Geometry check sheet. Reference: the model listing, model coordinates, mm. A direction names the side the tool comes from. Coordinates: 2 decimals unless noted, no trailing zeros. Loops run counter-clockwise (first coordinate to the right, second up) from the corner with the lowest first, then second, coordinate; pieces in that order, holes last. Notation, with made-up numbers: (-9, 30.25) - (2, 30.25) arc R27 ccw to (2, 54.25) - close; hole circle Ø6 at (87, 86.5). An arc over 180 degrees is marked (long way). Write item = value, one per line. Start each with the question number.
from build123d import *

# Parameters (mm, degrees)
SKETCH1_W              = 15
SKETCH1_H              = 15
SKETCH1_W_2            = 12
SKETCH1_H_2            = 12
EXTRUDE_THIN1_DEPTH    = 235
CUT_EXTRUDE1_OUTLINE_R = 1.5
CUT_EXTRUDE1_DEPTH     = 15
SKETCH3_R              = 1.5
CUT_EXTRUDE2_DEPTH     = 236.95550428


# Read off the part's stored shape, not the designer's step: Cut-Extrude1
with BuildPart() as part:
    # Sketch1 → Extrude-Thin1 (new body)
    with BuildSketch(Plane(origin=(0, 0, 0), x_dir=(1, 0, 0), z_dir=(0, 1, 0))):
        with Locations((7.5, 7.5)):
            Rectangle(SKETCH1_W, SKETCH1_H)
        with Locations((7.5, 7.5)):
            Rectangle(SKETCH1_W_2, SKETCH1_H_2, mode=Mode.SUBTRACT)
    extrude(amount=EXTRUDE_THIN1_DEPTH)

    # Cut-Extrude1 outline → Cut-Extrude1 (cut)
    with BuildSketch(Plane.YZ):
        with Locations((15, -7.5)):
            Circle(CUT_EXTRUDE1_OUTLINE_R)
        with Locations((5, -7.5)):
            Circle(CUT_EXTRUDE1_OUTLINE_R)
        with Locations((220, -7.5)):
            Circle(CUT_EXTRUDE1_OUTLINE_R)
        with Locations((230, -7.5)):
            Circle(CUT_EXTRUDE1_OUTLINE_R)
    extrude(amount=CUT_EXTRUDE1_DEPTH, mode=Mode.SUBTRACT)

    # Sketch3 → Cut-Extrude2 (cut, through all)
    with BuildSketch(Plane(origin=(15, 0, 0), x_dir=(0, 0, -1), z_dir=(1, 0, 0))):
        with Locations((7.5, 80)):
            Circle(SKETCH3_R)
        with Locations((7.5, 70)):
            Circle(SKETCH3_R)
    extrude(amount=-CUT_EXTRUDE2_DEPTH, mode=Mode.SUBTRACT)


solid = part.part
(1) Sectioned sample at C-C on x = 10. Enter the section's corners in (y, z), plus the area to 3 significant figures.
(2) Tool access check on faces 1 (the face through (0, 116, -7)), 2 (the face through (7, 116, -1.5)). Record the directions out of +Z, -Z, +X, -X, +Y, -Y that give a thin tool (end or side, any length) a straight path to the whole face; none if there is none.
(3) Scan lines: line 1 (X direction, y = 50, z = -3.5); line 2 (Z direction, x = 13.95, y = 80); line 3 (Z direction, x = 2.5, y = 218.5). Record each from-to range of solid material in increasing order.
(4) Draft check along Z on faces 3 (the face through (13.5, 116, -7)), 4 (the face through (15, 116, -7)), 5 (the face through (7, 116, -15)), 6 (the face through (7, 116, 0)). Enter one of: pulls with the +Z half, pulls with the -Z half, needs draft (parallel to the pull), parting line crosses it, or undercut.
(5) Sectioned sample at A-A on z = -11. Enter the section's corners in (x, y).
(6) Sectioned sample at B-B on y = 96. Enter the section's corners in (x, z).
Working result:
q1.outline = (0, -15) - (235, -15) - (235, -13.5) - (0, -13.5) - close; (0, -1.5) - (235, -1.5) - (235, 0) - (0, 0) - close
q1.area = 705 mm2
q2.face_1 = +Z, -Z, -X, +Y, -Y
q2.face_2 = +Y, -Y
q3.line_1 = 0 to 1.5, 13.5 to 15
q3.line_2 = -15 to -9, -6 to 0
q3.line_3 = -15 to -13.5, -1.5 to 0
q4.face_3 = undercut
q4.face_4 = needs draft
q4.face_5 = pulls with the -Z half
q4.face_6 = pulls with the +Z half
q5.outline = (0, 0) - (1.5, 0) - (1.5, 235) - (0, 235) - close; (13.5, 0) - (15, 0) - (15, 235) - (13.5, 235) - close
q6.outline = (0, -15) - (15, -15) - (15, 0) - (0, 0) - close; hole (1.5, -13.5) - (13.5, -13.5) - (13.5, -1.5) - (1.5, -1.5) - close
